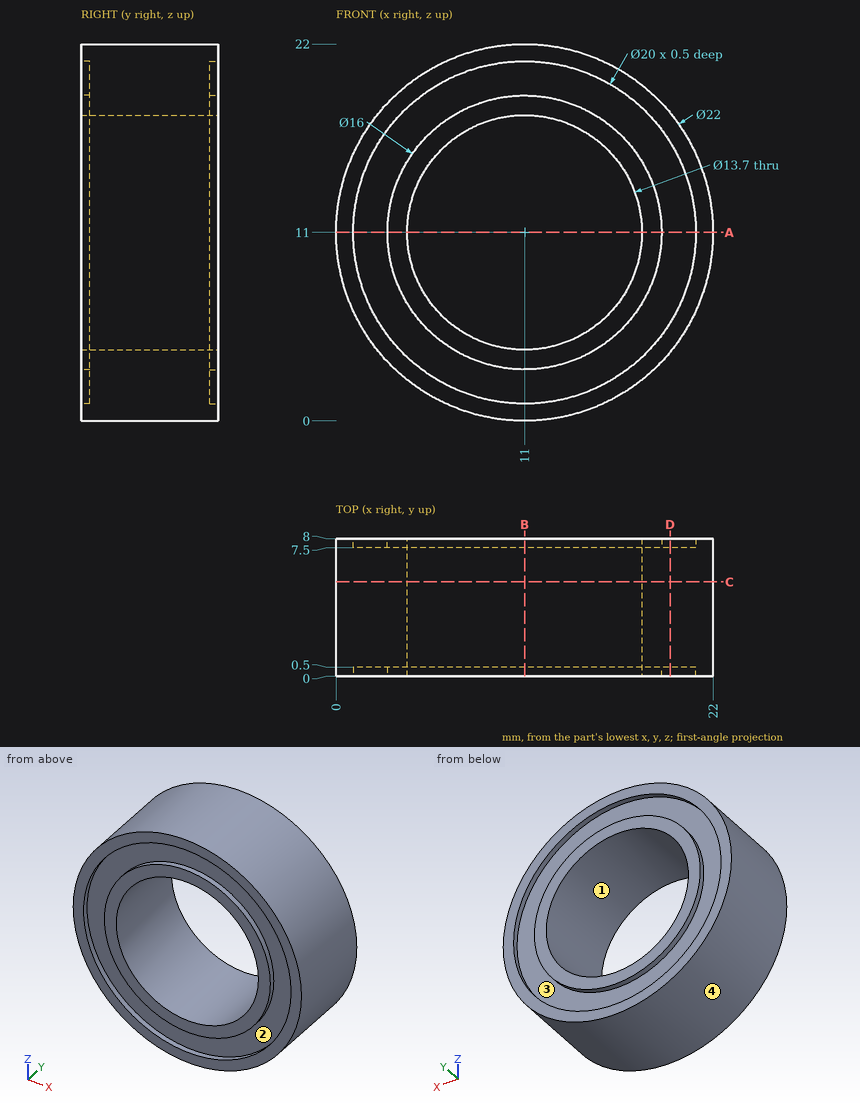
The drawing under review shows one solid part. Ordinate dimensions are in mm from its lowest x, y, z. A direction names the side the tool comes from. Round coordinates to 2 decimals unless told otherwise and drop trailing zeros. Order: outer loops, then holes, each group sorted by start corner. A loop starts at its lowest first (then second) coordinate and runs counter-clockwise, first axis right, second up. Notation, with made-up numbers: (15.25, 34.25) -> (49.25, 34.25) arc R28 ccw to (49.25, 53.25) -> close; hole circle Ø11 at (-18.5, 59). An arc over 180 degrees is marked (long way). Use a Markdown table: item, result.
Item 1: Take a section at A-A (z = 11). State the section outline as (x, y) points.
Resolved:
| item | result |
|---|---|
| outline | (0, 0) -> (1, 0) -> (1, 0.5) -> (3, 0.5) -> (3, 0) -> (4.15, 0) -> (4.15, 8) -> (3, 8) -> (3, 7.5) -> (1, 7.5) -> (1, 8) -> (0, 8) -> close; (17.85, 0) -> (19, 0) -> (19, 0.5) -> (21, 0.5) -> (21, 0) -> (22, 0) -> (22, 8) -> (21, 8) -> (21, 7.5) -> (19, 7.5) -> (19, 8) -> (17.85, 8) -> close |
Item 2: Take a section at D-D (x = 19.5). State the section outline as (y, z) points, plus the area to 3 significant figures.
Resolved:
| item | result |
|---|---|
| outline | (0, 4.02) -> (8, 4.02) -> (8, 5.73) -> (7.5, 5.73) -> (7.5, 16.27) -> (8, 16.27) -> (8, 17.98) -> (0, 17.98) -> (0, 16.27) -> (0.5, 16.27) -> (0.5, 5.73) -> (0, 5.73) -> close |
| area | 101 mm² |
Item 3: Machinability: for the marked faces 1 and 2, which of the approach directions +Z, -Z, +X, -X, +Y, -Y give a long, thin tool a straight path to every point of the face, cutting with its end or side? Answer none if there is none.
Resolved:
| item | result |
|---|---|
| face 1 | +Y, -Y |
| face 2 | -Y |
Item 4: For pin 1 (4 mm diameter, centred on y = 4.5, z = 15, fed in from +X); pin 2 (12 mm diameter, centred on x = 11, z = 11, fed in from -Y), all flat-tipped, find the tip position at first contact; note any pin that passes through.
Resolved:
| item | result |
|---|---|
| pin 1 | stops at x = 21.82 |
| pin 2 | passes through |
Item 5: Draft analysis for pull direction Z (two halves, no side actions). For the marked faces 3 and 4, state which applies: +Z half, -Z half, draft (parallel to the pull), parting line (faces both ways), or undercut.
Resolved:
| item | result |
|---|---|
| face 3 | undercut |
| face 4 | parting line |
Item 6: For line 1 along X through (y, z) = (7.7, 11); line 2 along X through (y, z) = (4.5, 11), list the stretches that pass through material, from the lowest coordinate up. Write a range as [from, to].
Resolved:
| item | result |
|---|---|
| line 1 | x = [0, 1], [3, 4.15], [17.85, 19], [21, 22] |
| line 2 | x = [0, 4.15], [17.85, 22] |
Item 7: Take a section at C-C (y = 5.5). State the section outline as (x, z) points.
Resolved:
| item | result |
|---|---|
| outline | circle Ø22 at (11, 11); hole circle Ø13.7 at (11, 11) |
Item 8: Take a section at B-B (x = 11). State the section outline as (y, z) points, plus the area to 3 significant figures.
Resolved:
| item | result |
|---|---|
| outline | (0, 0) -> (8, 0) -> (8, 1) -> (7.5, 1) -> (7.5, 3) -> (8, 3) -> (8, 4.15) -> (0, 4.15) -> (0, 3) -> (0.5, 3) -> (0.5, 1) -> (0, 1) -> close; (0, 17.85) -> (8, 17.85) -> (8, 19) -> (7.5, 19) -> (7.5, 21) -> (8, 21) -> (8, 22) -> (0, 22) -> (0, 21) -> (0.5, 21) -> (0.5, 19) -> (0, 19) -> close |
| area | 62.4 mm² |
